Input: part model. Units: mm. Frame: model coordinates. Round coordinates to 2 decimals unless told otherwise and drop trailing zeros. Order: outer loops, then holes, each group sorted by start corner. A loop starts at its lowest first (then second) coordinate and runs counter-clockwise, first axis right, second up. Notation, with made-up numbers: M 82,8 L 122,8 A38 cw 122,47 Z; hole C 6,-36.5 d11. An arc over 180 degrees is marked long. One line per question, with ' | ' between items.
```python
from build123d import *

# Parameters (mm, degrees)
EXTRUDE_1_DEPTH     = 655
SKETCH_2_R          = 2.15
CUT_EXTRUDE_1_DEPTH = 3.9


with BuildPart() as part:
    # ｽｹｯﾁ1 → ﾎﾞｽ - 押し出し1 (new body)
    with BuildSketch(Plane.XY):
        Polygon((4, -2.5), (3, 0), (0, 0), (0, -3.9), (5.05, -3.9), (6.65, -5), (7.65, -5), (7.65, -2.5), align=None)
        Polygon((0, -3.9), (0, 0), (-3, 0), (-4, -2.5), (-7.65, -2.5), (-7.65, -5), (-6.65, -5), (-5.05, -3.9), align=None)
    extrude(amount=EXTRUDE_1_DEPTH)

    # ｽｹｯﾁ2 → ｶｯﾄ - 押し出し1 (cut)
    with BuildSketch(Plane(origin=(0, 0, 0), x_dir=(1, 0, 0), z_dir=(0, 1, 0))):
        with Locations(Location((0, -7.5, 0), (0, 0, 270))):
            Circle(SKETCH_2_R)
        with Locations(Location((0, -647.5, 0), (0, 0, 270))):
            Circle(SKETCH_2_R)
    extrude(amount=-CUT_EXTRUDE_1_DEPTH, mode=Mode.SUBTRACT)


solid = part.part
```
Item 1: Section query A-A, the plane y = -1.05. Return loops of the section in (x, z).
Report:
outline: M -3.42,0 L 3.42,0 L 3.42,655 L -3.42,655 Z; hole C 0,7.5 d4.3; hole C 0,647.5 d4.3
Item 2: First-contact query: pin 1 (2 mm diameter, centred on x = 4, z = 413.5, fed in from -Y); pin 2 (1.1 mm diameter, centred on x = 5, z = 266.5, fed in from +Y). Flat tips, straight axial feed; report the tip coordinate or a pass-through.
Report:
pin 1: y = -3.9 | pin 2: y = -2.5
Item 3: Line query: line 1 along Z through (x, y) = (-1, -0.75); line 2 along X through (y, z) = (-2.35, 7.5); line 3 along X through (y, z) = (-2.55, 7.5). Output: solid intervals per line, ascending. Write a range as from..to.
Report:
line 1: 0..5.6, 9.4..645.6, 649.4..655 | line 2: -3.94..-2.15, 2.15..3.94 | line 3: -7.65..-2.15, 2.15..7.65
Item 4: Section query B-B, the plane z = 494.5. Return loops of the section in (x, y).
Report:
outline: M -7.65,-5 L -6.65,-5 L -5.05,-3.9 L 5.05,-3.9 L 6.65,-5 L 7.65,-5 L 7.65,-2.5 L 4,-2.5 L 3,0 L -3,0 L -4,-2.5 L -7.65,-2.5 Z
